Source: CAD feature listing. Evaluate the final solid. Frame: model axes, mm. A direction names the side the tool comes from. Coordinates: 2 decimals unless noted, no trailing zeros. Order: outer loops, then holes, each group sorted by start corner. A loop starts at its lowest first (then second) coordinate and runs counter-clockwise, first axis right, second up. Notation, with made-up numbers: (55.5, 3) -> (94.5, 3) arc R23 ccw to (94.5, 27) -> close; hole circle Ø1 at (-15, 3). An arc over 180 degrees is marked (long way). Write item = value, one per line. Start each with the question number.
Item 1: Ray query, line 1 along X through (y, z) = (55, -28); line 2 along Y through (x, z) = (-66, 2); line 3 along X through (y, z) = (52, -6.5). Return the intervals inside material, ascending. Write a range as [from, to].
Item 2: Contact query for flat-ended pins moving along their axis: pin 1 (1 mm diameter, centred on x = -2, y = 5, fed in from -Z); pin 2 (5.5 mm diameter, centred on x = 75.5, y = 48, fed in from -Z); pin 3 (10 mm diameter, centred on x = -54, z = -25, fed in from +Y); pin 4 (0.6 mm diameter, centred on x = 64, y = 20.5, fed in from -Z). Output: stop coordinate, or through.
Item 3: Section query B-B (z = -24.5). Count the separate pieces of the cut face and the enclosed holes in it, then the cut area to 3 significant figures.
Item 4: Mould query, pull axis Y, two halves, no side actions, for faces 1 (the flat face through (-65, 21, -32.8)), 2 (the cylindrical face through (-73.43, 65.42, 0.34)). Classes: released by +Y, released by -Y, zero draft, split by the parting line, or undercut.
Item 5: Section query C-C (x = -30.5). Output: boundary loops of the cut face in (y, z), then the cut area to 3 significant figures.
Item 6: Set-up query: faces 3 (the cylindrical face through (73.34, 65.42, 0.43)), 4 (the flat face through (77, 35, -18)), 5 (the cylindrical face through (71.797, 62.321, -1.141)). Return all of +Z, -Z, +X, -X, +Y, -Y with unobstructed straight access to the full face (end or side cutting, diameter ignored); none if empty.
Item 7: Section query A-A (y = 35). Output: boundary loops of the cut face in (x, z).
```python
from build123d import *

# Parameters (mm, degrees)
SKETCH002_R     = 1.5
POCKET_DEPTH    = 23.001
SKETCH003_R     = 4
PAD_DEPTH       = 35
SKETCH004_R     = 1
POCKET001_DEPTH = 10


with BuildPart() as part:
    # AdditivePipe: sweep along a path in Sketch001
    with BuildLine(Plane.XZ) as additivepipe_path:
        Line((-73, -18), (-73, -4))
        ThreePointArc((-73, -4), (-71.828427, -1.171573), (-69, 0))
        Line((-69, 0), (0, 0))
        Line((0, 0), (69, 0))
        ThreePointArc((69, 0), (71.828427, -1.171573), (73, -4))
        Line((73, -4), (73, -18))
    # Sketch → AdditivePipe (sweep)
    with BuildSketch(Plane.YZ):
        Polygon((0, 5), (70, 5), (70, 0), (67, 0), (67, 2.2), (63.8, 2.2), (63.8, 0), (60.8, 0), (60.8, 2.2), (9.2, 2.2), (9.2, 0), (6.2, 0), (6.2, 2.2), (3, 2.2), (3, 0), (0, 0), align=None)
    sweep(path=additivepipe_path.line)

    # Sketch002 (on Face35 of AdditivePipe) → Pocket (cut, through all)
    with BuildSketch(Plane(origin=(0, 0, 5), x_dir=(0, -1, 0), z_dir=(0, 0, 1))):
        with Locations((-35, -64)):
            Circle(SKETCH002_R)
        with Locations((-35, 64)):
            Circle(SKETCH002_R)
        with Locations((-35, 0)):
            Circle(SKETCH002_R)
    extrude(amount=-POCKET_DEPTH, mode=Mode.SUBTRACT)

    # Sketch003 (on Face43 of Pocket) → Pad (join)
    with BuildSketch(Plane.YX.offset(-2.2)):
        with Locations((20, 64)):
            Circle(SKETCH003_R)
        with Locations((55, 64)):
            Circle(SKETCH003_R)
        with Locations((20, 0)):
            Circle(SKETCH003_R)
        with Locations((55, 0)):
            Circle(SKETCH003_R)
        with Locations((20, -64)):
            Circle(SKETCH003_R)
        with Locations((55, -64)):
            Circle(SKETCH003_R)
    extrude(amount=PAD_DEPTH)

    # Sketch004 (on Face88 of Pad) → Pocket001 (cut)
    with BuildSketch(Plane.YX.offset(32.8)):
        with Locations((20, 64)):
            Circle(SKETCH004_R)
        with Locations((55, 64)):
            Circle(SKETCH004_R)
        with Locations((20, 0)):
            Circle(SKETCH004_R)
        with Locations((55, 0)):
            Circle(SKETCH004_R)
        with Locations((20, -64)):
            Circle(SKETCH004_R)
        with Locations((55, -64)):
            Circle(SKETCH004_R)
    extrude(amount=-POCKET001_DEPTH, mode=Mode.SUBTRACT)


solid = part.part
```
Computed:
q1.line_1 = [-68, -65], [-63, -60], [-4, -1], [1, 4], [60, 63], [65, 68]
q1.line_2 = [0, 3], [6.2, 9.2], [16.54, 23.46], [51.54, 58.46], [60.8, 63.8], [67, 70]
q1.line_3 = [-78, -75.2], [-66.65, -61.35], [-2.65, 2.65], [61.35, 66.65], [75.2, 78]
q2.pin_1 = 2.2
q2.pin_2 = -18
q2.pin_3 = through
q2.pin_4 = -22.8
q3.separate_pieces = 6
q3.enclosed_holes = 6
q3.area = 283 mm^2
q4.face_1 = zero draft
q4.face_2 = undercut
q5.outline = (0, 0) -> (3, 0) -> (3, 2.2) -> (6.2, 2.2) -> (6.2, 0) -> (9.2, 0) -> (9.2, 2.2) -> (60.8, 2.2) -> (60.8, 0) -> (63.8, 0) -> (63.8, 2.2) -> (67, 2.2) -> (67, 0) -> (70, 0) -> (70, 5) -> (0, 5) -> close
q5.area = 222 mm^2
q6.face_3 = -Z
q6.face_4 = -Z, +X, +Y, -Y
q6.face_5 = -Z, +Y, -Y
q7.outline = (-78, -18) -> (-75.2, -18) -> (-75.2, -4) arc R6.2 cw to (-69, 2.2) -> (-65.5, 2.2) -> (-65.5, 5) -> (-69, 5) arc R9 ccw to (-78, -4) -> close; (-62.5, 2.2) -> (-1.5, 2.2) -> (-1.5, 5) -> (-62.5, 5) -> close; (1.5, 2.2) -> (62.5, 2.2) -> (62.5, 5) -> (1.5, 5) -> close; (65.5, 2.2) -> (69, 2.2) arc R6.2 cw to (75.2, -4) -> (75.2, -18) -> (78, -18) -> (78, -4) arc R9 ccw to (69, 5) -> (65.5, 5) -> close
